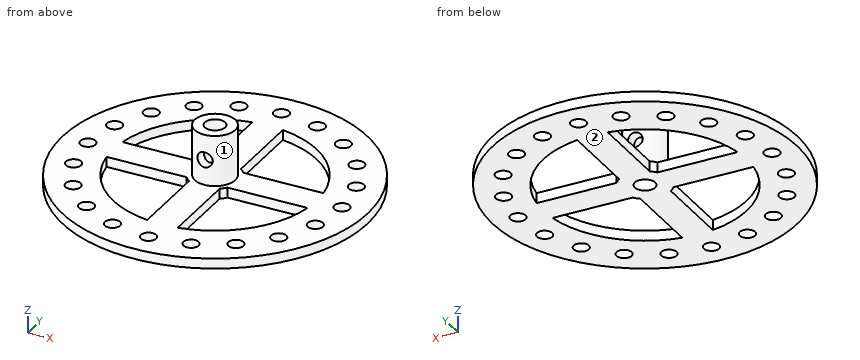
Autodesk Fusion 360 part; units mm, degrees
sketch "スケッチ1" plane through (0, 0, 0) normal (0, 0, 1) x (1, 0, 0)
  circle A0 centre (0, 0) radius 30
  circle A1 centre (0, 0) radius 20
  circle A2 centre (0, 0) radius 5
  circle A3 centre (0, 25) radius 1.5
  line L0 (-3, 4) -> (-3, 19.7737)
  line L1 (3, 4) -> (3, 19.7737)
  line L2 (-4, 3) -> (-19.7737, 3)
  line L3 (-4, -3) -> (-19.7737, -3)
  line L4 (-3, -4) -> (-3, -19.7737)
  line L5 (3, -4) -> (3, -19.7737)
  line L6 (4, -3) -> (19.7737, -3)
  line L7 (4, 3) -> (19.7737, 3)
  circle A4 centre (-7.7254, 23.7764) radius 1.5
  circle A5 centre (-14.6946, 20.2254) radius 1.5
  circle A6 centre (-20.2254, 14.6946) radius 1.5
  circle A7 centre (-23.7764, 7.7254) radius 1.5
  circle A8 centre (-25, 0) radius 1.5
  circle A9 centre (-23.7764, -7.7254) radius 1.5
  circle A10 centre (-20.2254, -14.6946) radius 1.5
  circle A11 centre (-14.6946, -20.2254) radius 1.5
  circle A12 centre (-7.7254, -23.7764) radius 1.5
  circle A13 centre (0, -25) radius 1.5
  circle A14 centre (7.7254, -23.7764) radius 1.5
  circle A15 centre (14.6946, -20.2254) radius 1.5
  circle A16 centre (20.2254, -14.6946) radius 1.5
  circle A17 centre (23.7764, -7.7254) radius 1.5
  circle A18 centre (25, 0) radius 1.5
  circle A19 centre (23.7764, 7.7254) radius 1.5
  circle A20 centre (20.2254, 14.6946) radius 1.5
  circle A21 centre (14.6946, 20.2254) radius 1.5
  circle A22 centre (7.7254, 23.7764) radius 1.5
  dimension "d2" = 360
  dimension "d4" = 360
extrude "押し出し1" add sketch "スケッチ1" along normal blind 2 contours A0 | A1 A2 L6 L7 | A1 A2 L0 L1 | A2 | A1 A2 L4 L5 | A1 A2 L2 L3
sketch "スケッチ2" plane through (0, 0, 2) normal (0, 0, 1) x (-1, 0, 0)
  circle A0 centre (0, -25) radius 1.5
  circle A1 centre (7.7254, 23.7764) radius 1.5
  circle A2 centre (14.6946, -20.2254) radius 1.5
  circle A3 centre (23.7764, -7.7254) radius 1.5
  circle A4 centre (14.6946, 20.2254) radius 1.5
  circle A5 centre (25, 0) radius 1.5
  circle A6 centre (20.2254, 14.6946) radius 1.5
  circle A7 centre (-7.7254, -23.7764) radius 1.5
  circle A8 centre (0, 0) radius 30
  arc A9 (-4, -3) -> (-3, -4) centre (0, 0) ccw
  line L0 (-3, -4) -> (-3, -19.7737)
  arc A10 (-19.7737, -3) -> (-3, -19.7737) centre (0, 0) ccw
  line L1 (-19.7737, -3) -> (-4, -3)
  line L2 (-3, 19.7737) -> (-3, 4)
  arc A11 (-3, 4) -> (-4, 3) centre (0, 0) ccw
  line L3 (-4, 3) -> (-19.7737, 3)
  arc A12 (-3, 19.7737) -> (-19.7737, 3) centre (0, 0) ccw
  circle A13 centre (-14.6946, 20.2254) radius 1.5
  circle A14 centre (-23.7764, -7.7254) radius 1.5
  line L4 (3, -19.7737) -> (3, -4)
  arc A15 (3, -4) -> (4, -3) centre (0, 0) ccw
  line L5 (4, -3) -> (19.7737, -3)
  arc A16 (3, -19.7737) -> (19.7737, -3) centre (0, 0) ccw
  line L6 (19.7737, 3) -> (4, 3)
  arc A17 (4, 3) -> (3, 4) centre (0, 0) ccw
  line L7 (3, 4) -> (3, 19.7737)
  arc A18 (19.7737, 3) -> (3, 19.7737) centre (0, 0) ccw
  circle A19 centre (-25, 0) radius 1.5
  circle A20 centre (-23.7764, 7.7254) radius 1.5
  circle A21 centre (23.7764, 7.7254) radius 1.5
  circle A22 centre (-14.6946, -20.2254) radius 1.5
  circle A23 centre (-20.2254, -14.6946) radius 1.5
  circle A24 centre (7.7254, -23.7764) radius 1.5
  circle A25 centre (-20.2254, 14.6946) radius 1.5
  circle A26 centre (0, 25) radius 1.5
  circle A27 centre (-7.7254, 23.7764) radius 1.5
  circle A28 centre (20.2254, -14.6946) radius 1.5
  circle A29 centre (0, 0) radius 2
  circle A30 centre (0, 0) radius 4
extrude "押し出し2" add sketch "スケッチ2" along normal blind 6 contours A30
extrude "押し出し3" cut 1 faces at (-0.4157, -0.5212, 2) along direction (0, 0, -1) blind 2
extrude "押し出し4" add 1 faces at (-3.311, 0.2981, 8) along direction (0, 0, 1) blind 4
ref_plane "作業平面1" through (0, 0, 6) normal (0, 1, 0) x (0, 0, 1)
sketch "スケッチ3" plane through (0, 0, 0) normal (0, 1, 0) x (1, 0, 0)
  circle A0 centre (0, -7) radius 1.5
extrude "押し出し5" cut sketch "スケッチ3" along normal blind 4 and the other way blind 4
Can you work these out from the model? Positions are in its coordinate system, mm. Face numbers are marked on the shaded views. A direction names the side the tool comes from. Coordinates: 2 decimals unless noted, no trailing zeros. Order: outer loops, then holes, each group sorted by start corner. A loop starts at its lowest first (then second) coordinate and runs counter-clockwise, first axis right, second up. Notation, with made-up numbers: (13.5, 28) -> (63.5, 28) arc R16 cw to (63.5, 50) -> close; hole circle Ø2 at (82.25, -31.75). An arc over 180 degrees is marked (long way). Use one line per item in the form item = value.
Q1. Which directions (+Z, -Z, +X, -X, +Y, -Y) give clear straight access to the entire face, cutting with the end or side of a thin tool? Please do the marked faces 1 and 2.
From the geometry:
face_1 = +Z
face_2 = -Z, +X, -X, +Y, -Y
Q2. Imagine slicing it at A-A, the plane x = 0. List the corners of the cut face in (y, z) for me, then the cut area to 3 significant figures.
From the geometry:
outline = (-30, 0) -> (-26.5, 0) -> (-26.5, 2) -> (-30, 2) -> close; (-23.5, 0) -> (-2, 0) -> (-2, 5.5) -> (-4, 5.5) -> (-4, 2) -> (-23.5, 2) -> close; (-4, 8.5) -> (-2, 8.5) -> (-2, 12) -> (-4, 12) -> close; (2, 0) -> (23.5, 0) -> (23.5, 2) -> (4, 2) -> (4, 5.5) -> (2, 5.5) -> close; (2, 8.5) -> (4, 8.5) -> (4, 12) -> (2, 12) -> close; (26.5, 0) -> (30, 0) -> (30, 2) -> (26.5, 2) -> close
area = 128 mm²
Q3. I need wall thicknesses on L1, parallel to Y at x = 0, z = 1.55; L2, parallel to Y at x = 1, z = 0.75. Which ranges of each line are inside material? Lowest first, please.
From the geometry:
L1 = -30 to -26.5, -23.5 to -2, 2 to 23.5, 26.5 to 30
L2 = -29.98 to -26.12, -23.88 to -1.73, 1.73 to 23.88, 26.12 to 29.98
Q4. Will these pins go through, and if not, where does the flat tip stop? P1, Ø1, axis at x = 14, z = 0.5, coming from the -Y side; P2, Ø2.5, axis at x = -25, y = 0, coming from the -Z side; P3, Ø2, axis at y = -0.5, z = 6, coming from the -X side; P4, Ø4, axis at x = 0, z = 7, coming from the +Y side.
From the geometry:
P1 = -26.79
P2 = through
P3 = -4
P4 = 4
Q5. Imagine slicing it at C-C, the plane z = 7. List the corners of the cut face in (x, y) for me, then the cut area to 3 significant figures.
From the geometry:
outline = (-1.5, -3.71) -> (-1.5, -1.32) arc R2 cw to (-1.5, 1.32) -> (-1.5, 3.71) arc R4 ccw to start; (1.5, -3.71) arc R4 ccw to (1.5, 3.71) -> (1.5, 1.32) arc R2 cw to (1.5, -1.32) -> close
area = 25.0 mm²
Q6. Imagine slicing it at D-D, the plane x = -10. List the corners of the cut face in (y, z) for me, then the cut area to 3 significant figures.
From the geometry:
outline = (-28.28, 0) -> (-17.32, 0) -> (-17.32, 2) -> (-28.28, 2) -> close; (-3, 0) -> (3, 0) -> (3, 2) -> (-3, 2) -> close; (17.32, 0) -> (28.28, 0) -> (28.28, 2) -> (17.32, 2) -> close
area = 55.9 mm²
Q7. Imagine slicing it at B-B, the plane y = 21. List the corners of the cut face in (x, z) for me.
From the geometry:
outline = (-21.42, 0) -> (-15.98, 0) -> (-15.98, 2) -> (-21.42, 2) -> close; (-13.41, 0) -> (13.41, 0) -> (13.41, 2) -> (-13.41, 2) -> close; (15.98, 0) -> (21.42, 0) -> (21.42, 2) -> (15.98, 2) -> close
